CAD build for the part. Positions are in the model's coordinates, mm. Face numbers are marked on the shaded views. A direction names the side the tool comes from. Give positions to 0.01 mm unless a question says otherwise; leave off trailing zeros. Write each loop counter-clockwise with the first axis right and the second up, starting at its lowest first coordinate (ties: lowest second). Pieces come first, ordered by that corner, then holes. Notation, with made-up numbers: (80.25, -37.75) - (103.25, -37.75) arc R16 cw to (103.25, -29.75) - close; hole circle Ø7 at (-1, 11). An arc over 180 degrees is marked (long way). Write item = value, one per line. Start each with the question number.
```python
from build123d import *

# Parameters (mm, degrees)
F0_R           = 17.5
F1_DEPTH       = 30
F0_R_2         = 22.5
F2_DEPTH       = 5
F4_D           = 7
F4_DEPTH       = 20
F4_CBORE_D     = 14
F4_CBORE_DEPTH = 3
F4_TIP         = 2.1030121666
F5_SIZE        = 0.5


with BuildPart() as f1:
    # F0 (on Front) → F1 (new body)
    with BuildSketch(Plane.XZ):
        Circle(F0_R)
    extrude(amount=F1_DEPTH)

    # F0 (on Front) → F2 (join)
    with BuildSketch(Plane.XZ):
        Circle(F0_R_2)
        Circle(F0_R, mode=Mode.SUBTRACT)
    extrude(amount=F2_DEPTH)

    # F4
    with Locations(Plane(origin=(0, 0, 0), x_dir=(-1, 0, 0), z_dir=(0, 1, 0))):
        with Locations((0, 0)):
            CounterBoreHole(F4_D / 2, F4_CBORE_D / 2, F4_CBORE_DEPTH, depth=F4_DEPTH)
            with Locations((0, 0, -(F4_DEPTH + F4_TIP / 2))):  # 118° drill point
                Cone(0, F4_D / 2, F4_TIP, mode=Mode.SUBTRACT)

    # F5
    f5_edges = [f1.edges().sort_by_distance(p)[0] for p in [
        (-17.5, -30, 0),
        (-22.5, -5, 0),
    ]]
    chamfer(f5_edges, length=F5_SIZE)


solid = f1.part
```
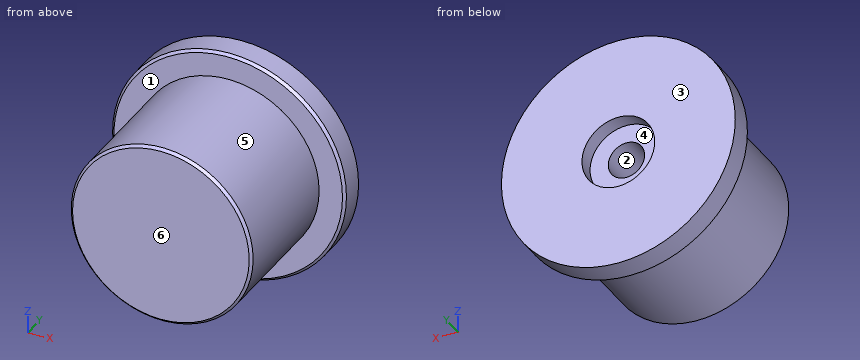
1. Pin check, flat tips, straight feed: pin 1 Ø10 at (y, z) = (-16.5, 12.5) entering from +X; pin 2 Ø2 at (x, y) = (-17, -24.5) entering from -Z; pin 3 Ø6 at (y, z) = (-13.5, 14.5) entering from -X. Stop position of each tip, or through.
2. Mould opens along Z. For the marked faces 4, 5 and 6 say: +Z half, -Z half, draft (parallel to the pull), parting line (faces both ways), or undercut.
3. Cut at A-A (y = -2.25). Give the cut face in (x, z), then the cut area to 3 significant figures.
4. Cut at B-B (y = -14). Give the cut face in (x, z).
5. Wall check: line 1 along Z through (x, y) = (0, -1.15); line 2 along Y through (x, z) = (16.5, 7); line 3 along Z through (x, y) = (-8, -3.75). Give the ranges that are in metal, low to high.
6. Tool access for the marked faces 1, 2 and 3: list every direction of +Z, -Z, +X, -X, +Y, -Y with a clear straight run to the whole face (end or side of a thin tool).
Output:
q1.pin_1 = 15.81
q1.pin_2 = -7.09
q1.pin_3 = -13.19
q2.face_4 = undercut
q2.face_5 = parting line
q2.face_6 = draft
q3.outline = circle Ø45 at (0, 0); hole circle Ø14 at (0, 0)
q3.area = 1,440 mm2
q4.outline = circle Ø35 at (0, 0); hole circle Ø7 at (0, 0)
q5.line_1 = -22.5 to -7, 7 to 22.5
q5.line_2 = -5 to 0
q5.line_3 = -21.03 to 21.03
q6.face_1 = -Y
q6.face_2 = +Y
q6.face_3 = +Z, -Z, +X, -X, +Y
